from build123d import *

# Parameters (mm, degrees)
SKETCH1_W           = 107
SKETCH1_H           = 95
SKETCH1_W_2         = 6.717391304
SKETCH1_H_2         = 79
SKETCH1_W_3         = 6.717391305
SKETCH1_W_4         = 15
SKETCH1_H_3         = 34
BOSS_EXTRUDE1_DEPTH = 4
CUT_EXTRUDE1_DEPTH  = 2
SKETCH5_W           = 2.000809174
SKETCH5_H           = 34
BOSS_EXTRUDE3_DEPTH = 8
SKETCH6_W           = 2
SKETCH6_H           = 22.102752069
CUT_EXTRUDE2_DEPTH  = 2
SKETCH7_W           = 1.989121342
SKETCH7_H           = 2
BOSS_EXTRUDE4_DEPTH = 30


with BuildPart() as part:
    # Sketch1 → Boss-Extrude1 (new body)
    # profile 1 of 2: a face of its own
    with BuildSketch(Plane.XY):
        with Locations((-0.188618926, -8.710358056)):
            Rectangle(SKETCH1_W, SKETCH1_H)
        with Locations((-40.699488491, -8.710358056)):
            Rectangle(SKETCH1_W_2, SKETCH1_H_2, mode=Mode.SUBTRACT)
        with Locations((-27.328779255, -8.658557904)):
            Rectangle(SKETCH1_W_2, SKETCH1_H_2, mode=Mode.SUBTRACT)
        with Locations((-13.692855398, -8.457629635)):
            Rectangle(SKETCH1_W_2, SKETCH1_H_2, mode=Mode.SUBTRACT)
        with Locations((0.382489646, -8.294414238)):
            Rectangle(SKETCH1_W_3, SKETCH1_H_2, mode=Mode.SUBTRACT)
        with Locations((13.672826098, -8.166203861)):
            Rectangle(SKETCH1_W_2, SKETCH1_H_2, mode=Mode.SUBTRACT)
        with Locations((27.177523355, -8.09026595)):
            Rectangle(SKETCH1_W_2, SKETCH1_H_2, mode=Mode.SUBTRACT)
        with Locations((40.840153453, -8.266624041)):
            Rectangle(SKETCH1_W_2, SKETCH1_H_2, mode=Mode.SUBTRACT)
    # profile 2 of 2: a face of its own
    with BuildSketch(Plane.XY):
        with Locations((-61.188618926, -39.210358056)):
            Rectangle(SKETCH1_W_4, SKETCH1_H_3)
    extrude(amount=BOSS_EXTRUDE1_DEPTH)

    # Sketch3 → Cut-Extrude1 (cut)
    with BuildSketch(Plane.XY.offset(4)):
        Polygon((51.311381074, -54.210358056), (51.311381074, 36.789641944), (-51.688618926, 36.789641944), (-51.688618926, -24.210358056), (-66.688618926, -24.210358056), (-66.688618926, -54.210358056), align=None)
    extrude(amount=-CUT_EXTRUDE1_DEPTH, mode=Mode.SUBTRACT)

    # Sketch5 → Boss-Extrude3 (add)
    with BuildSketch(Plane.XY.offset(4)):
        with Locations((-67.688214339, -39.210358056)):
            Rectangle(SKETCH5_W, SKETCH5_H)
    extrude(amount=BOSS_EXTRUDE3_DEPTH)

    # Sketch6 → Cut-Extrude2 (cut)
    with BuildSketch(Plane.XY.offset(4)):
        with Locations((52.311381074, 13.925496341)):
            Rectangle(SKETCH6_W, SKETCH6_H)
    extrude(amount=-CUT_EXTRUDE2_DEPTH, mode=Mode.SUBTRACT)

    # Sketch7 → Boss-Extrude4 (add)
    with BuildSketch(Plane.XZ.offset(24.210358056)):
        with Locations((-52.693548431, 3)):
            Rectangle(SKETCH7_W, SKETCH7_H)
    extrude(amount=BOSS_EXTRUDE4_DEPTH)


solid = part.part
Can you work these out from the model? Positions are in its coordinate system, mm. A direction names the side the tool comes from. Coordinates: 2 decimals unless noted, no trailing zeros. Loops run counter-clockwise (first coordinate to the right, second up) from the corner with the lowest first, then second, coordinate; pieces in that order, holes last. Notation, with made-up numbers: (23, -10) - (43, -10) arc R9 ccw to (43, -1) - close; hole circle Ø10 at (65, -4.75). An arc over 180 degrees is marked (long way). Answer as a JSON object with one key per item and string values. Group by question number.
Item 1: On a 3-axis mill with a long thin cutter (end or side, diameter ignored), from which of +Z, -Z, +X, -X, +Y, -Y can I reach the whole of each face in a straight line? I mean faces 1 (the face through (-66.688, -39, 8)), 2 (the face through (-63, -22.21, 3)), 3 (the face through (-1, 38.79, 2)). Say none if no direction works.
Item 2: If we mould it in two halves opening along X, with no side actions, what happens to faces 4 (the face through (-53.689, 8, 2)), 5 (the face through (-12, -56.21, 3)), 6 (the face through (-60, -39, 2))? For each: released by +X, released by -X, zero draft, split by the parting line, or undercut.
Item 3: For pin 1 (0.6 mm diameter, centred on y = -1.5, z = 1, fed in from -X); pin 2 (8 mm diameter, centred on x = -9.5, y = 17, fed in from +Z); pin 3 (2.5 mm diameter, centred on y = -47, z = 6.5, fed in from +X), each with a flat end and sliding along its axis, tell me the tip position at first contact or that it passes through.
Item 4: If we section it at C-C (x = 21.5): List the corners of the cut face in (y, z) for me, plus the area to 3 significant figures.
Item 5: If we section it at A-A (y = 15): State how many separate pieces and enclosed holes the cut face has, plus the area to 3 significant figures.
Item 6: If we section it at D-D (z = 7.75): List the corners of the cut face in (x, y) for me.
Item 7: If I drill on L1, parallel to X at y = 31, z = 0.75; L2, parallel to Y at x = -6.5, z = 3; L3, parallel to Z at x = -53, y = -33, over which ranges is the centre line in solid material (lowest first)? Write a range as from..to.
Item 8: If we section it at B-B (x = -13.5): List the corners of the cut face in (y, z) for me, plus the area to 3 significant figures.
Returned:
{
 "1": {"face 1": "+Z, +X, +Y, -Y", "face 2": "+Z, -Z, -X, +Y", "face 3": "+Z, -Z, +X, -X, +Y"},
 "2": {"face 4": "released by -X", "face 5": "zero draft", "face 6": "undercut"},
 "3": {"pin 1": "stops at x = -53.69", "pin 2": "stops at z = 2", "pin 3": "stops at x = -66.69"},
 "4": {"outline": "(-56.21, 0) - (38.79, 0) - (38.79, 4) - (36.79, 4) - (36.79, 2) - (-54.21, 2) - (-54.21, 4) - (-56.21, 4) - close", "area": "198 mm²"},
 "5": {"separate pieces": "8", "enclosed holes": "0", "area": "124 mm²"},
 "6": {"outline": "(-68.69, -56.21) - (-66.69, -56.21) - (-66.69, -22.21) - (-68.69, -22.21) - close"},
 "7": {"L1": "x = -53.69..-17.05, -10.33..-2.98, 3.74..10.31, 17.03..23.82, 30.54..37.48, 44.2..53.31", "L2": "y = -56.21..-54.21, 36.79..38.79", "L3": "z = 0..4"},
 "8": {"outline": "(-56.21, 0) - (-47.96, 0) - (-47.96, 2) - (-54.21, 2) - (-54.21, 4) - (-56.21, 4) - close; (31.04, 0) - (38.79, 0) - (38.79, 4) - (36.79, 4) - (36.79, 2) - (31.04, 2) - close", "area": "40.0 mm²"}
}
